Autodesk Inventor part; units mm, degrees
ref_plane "YZ Plane" through (0, 0, 0) normal (1, 0, 0) x (0, 1, 0)
ref_plane "XZ Plane" through (0, 0, 0) normal (0, 1, 0) x (-1, 0, 0)
ref_plane "XY Plane" through (0, 0, 0) normal (0, 0, 1) x (1, 0, 0)
sketch "Sketch1" plane through (0, 0, 0) normal (0, 1, 0) x (-1, 0, 0)
  arc A0 (0, 6) -> (0, -6) centre (0, 0) ccw
  line L0 (0, 0) -> (-14.5, 0) construction
  line L1 (0, 6) -> (0, 12.5)
  line L2 (0, 12.5) -> (-14.5, 12.5)
  line L3 (0, -6) -> (0, -12.5)
  line L4 (0, -12.5) -> (-14.5, -12.5)
  line L5 (-14.5, 12.5) -> (-14.5, -12.5)
extrude "Extrusion1" add sketch "Sketch1" along normal blind 8
sketch "Sketch2" plane through (0, 8, 0) normal (0, 1, 0) x (1, 0, 0)
  line L0 (14.5, -12.5) -> (14.5, 12.5) construction
  line L1 (0, 12.5) -> (0, 6) construction
  line L2 (0, -6) -> (0, -12.5) construction
  point P0 (0, 0)
sketch "Sketch3" plane through (0, 0, -12.5) normal (-1, 0, 0) x (0, 0, 1)
  line L0 (0, 8) -> (6.5, 8) construction
  line L1 (3.25, 8) -> (3.25, 0) construction
  line L2 (25, 8) -> (0, 8) construction
  line L3 (18.5, 8) -> (25, 8) construction
  line L4 (21.75, 8) -> (21.75, 0) construction
  line L5 (12.5, 0) -> (12.5, 8) construction
  line L6 (25, 0) -> (25, 8) construction
  line L7 (25, 4) -> (0, 4) construction
  line L8 (0, 0) -> (0, 8) construction
  circle A0 centre (21.75, 4) radius 1.6
  circle A1 centre (3.25, 4) radius 1.6
  dimension "d8" = 3.2
  dimension "d9" = 3.2
extrude "Extrusion2" cut sketch "Sketch3" against normal through all
sketch "Sketch4" plane through (0, 8, 0) normal (0, 1, 0) x (1, 0, 0)
  point P0 (0, 0)
properties part number "Semi Cuscinetto"
Geometry: final body of the model. Coordinates: model frame, mm. Round coordinates to 2 decimals unless told otherwise and drop trailing zeros. Write each loop counter-clockwise with the first axis right and the second up, starting at its lowest first coordinate (ties: lowest second). Pieces come first, ordered by that corner, then holes.
Item 1: Section query C-C (x = 9.25). Return loops of the section in (y, z), plus the area to 3 significant figures.
Item 2: Section query B-B (z = 9.25). Return loops of the section in (x, y).
Item 3: Section query A-A (y = 4). Return loops of the section in (x, z), plus the area to 3 significant figures.
Item 4: Material intervals for L1, parallel to Y at x = 7.75, z = 9.25; L2, parallel to Z at x = 10, y = 3; L3, parallel to Z at x = 8.25, y = 3.25, sorted ascending.
Item 5: Mould query, pull axis Y, two halves, no side actions, for faces 1 (the face through (7, 4, -12.5)), 2 (the face through (9, 8, 0)), 3 (the face through (7.15, 4.07, -10.85)). Classes: +Y half, -Y half, draft (parallel to the pull), parting line (faces both ways), or undercut.
Item 6: Pin query (flat end, axial travel): P1, Ø2, axis at x = 3, z = 0.5, coming from the -Y side. Return the tip coordinate at first contact, or that it passes through.
Item 7: Section query D-D (y = 1.25). Return loops of the section in (x, z), plus the area to 3 significant figures.
Completed:
1. outline: (0, -12.5) - (8, -12.5) - (8, 12.5) - (0, 12.5) - close; hole circle Ø3.2 at (4, -9.25); hole circle Ø3.2 at (4, 9.25)
1. area: 184 mm2
2. outline: (0, 0) - (14.5, 0) - (14.5, 2.4) - (0, 2.4) - close; (0, 5.6) - (14.5, 5.6) - (14.5, 8) - (0, 8) - close
3. outline: (0, -12.5) - (14.5, -12.5) - (14.5, -10.85) - (0, -10.85) - close; (0, -7.65) - (14.5, -7.65) - (14.5, 7.65) - (0, 7.65) - (0, 6) arc R6 cw to (0, -6) - close; (0, 10.85) - (14.5, 10.85) - (14.5, 12.5) - (0, 12.5) - close
3. area: 213 mm2
4. L1: y = 0 to 2.4, 5.6 to 8
4. L2: z = -12.5 to -10.5, -8 to 8, 10.5 to 12.5
4. L3: z = -12.5 to -10.66, -7.84 to 7.84, 10.66 to 12.5
5. face 1: draft
5. face 2: +Y half
5. face 3: undercut
6. P1: passes through
7. outline: (0, -12.5) - (14.5, -12.5) - (14.5, 12.5) - (0, 12.5) - (0, 6) arc R6 cw to (0, -6) - close
7. area: 306 mm2
